Can you work these out from the model? Positions are in its coordinate system, mm. Round coordinates to 2 decimals unless told otherwise and drop trailing zeros. Write each loop counter-clockwise with the first axis right and the second up, starting at its lowest first coordinate (ties: lowest second). Pieces come first, ordered by that corner, then holes.
Q1. If we section it at C-C (y = 16): Please give me the cut outline in (x, z).
Q2. I'm going to push flat-ended pins straight in: pin 1 Ø0.7 at (y, z) = (25, 1) entering from +X; pin 2 Ø0.9 at (y, z) = (17.5, 1) entering from +X; pin 3 Ø1.6 at (x, z) = (-9, 1.5) entering from -Y. Where does each tip first touch, or does it pass through?
Q3. If we section it at A-A (y = -8): Give the number of separate pieces and of enclosed holes in the cut face, plus the area to 3 significant figures.
Q4. Please list where these lines run through material, in increasing order: line 1 along X through (y, z) = (23, 2.2); line 2 along X through (y, z) = (-12.5, 0.2); line 3 along X through (y, z) = (12.5, 2.95).
from build123d import *

# Parameters (mm, degrees)
SKETCH1_R           = 1.5
BOSS_EXTRUDE1_DEPTH = 3
SKETCH2_R           = 0.2
CUT_EXTRUDE1_DEPTH  = 51.771570482
CIRPATTERN1_COUNT   = 3
SKETCH3_R           = 8.5
CUT_EXTRUDE2_DEPTH  = 45.723637705
SKETCH4_R           = 1.5
SKETCH4_R_2         = 1.375
CUT_EXTRUDE3_DEPTH  = 45.723637705
CUT_EXTRUDE6_DEPTH  = 45.723637705
SKETCH10_R          = 1.6
BOSS_EXTRUDE3_DEPTH = 3
CUT_EXTRUDE7_DEPTH  = 46.118589611


with BuildPart() as part:
    # Sketch1 → Boss-Extrude1 (new body)
    with BuildSketch(Plane.XY):
        Polygon((8, 23), (8, 25.75), (10, 25.75), (10, 24.45), (15, 24.45), (15, 26.5), (10.5, 31), (-10.5, 31), (-15, 26.5), (-15, 24.45), (-10, 24.45), (-10, 25.75), (-8, 25.75), (-8, 23), (-8, 20.25), (-10, 20.25), (-10, 21.55), (-15, 21.55), (-15, 19.5), (-14, 18.5), (-14, 16.703779947), (-17.732948887, 10.238122813), (-21.465897773, 3.772465679), (-23.02146997, 2.874355653), (-24.387495374, 3.240381057), (-26.162847452, 2.215381057), (-23.662847452, -2.114745962), (-22.537014427, -1.464745962), (-21.537014427, -3.19679677), (-23.918584287, -4.57179677), (-26.300154147, -5.94679677), (-27.300154147, -4.214745962), (-26.174321123, -3.564745962), (-28.674321123, 0.765381057), (-30.4496732, -0.259618943), (-32.096787517, -6.40673326), (-21.596787517, -24.59326674), (-15.4496732, -26.240381057), (-13.674321123, -25.215381057), (-16.174321123, -20.885254038), (-17.300154147, -21.535254038), (-18.300154147, -19.80320323), (-15.918584287, -18.42820323), (-13.537014427, -17.05320323), (-12.537014427, -18.785254038), (-13.662847452, -19.435254038), (-11.162847452, -23.765381057), (-9.387495374, -22.740381057), (-9.02146997, -21.374355653), (-7.465897773, -20.476245627), (0, -20.476245627), (7.465897773, -20.476245627), (9.02146997, -21.374355653), (9.387495374, -22.740381057), (11.162847452, -23.765381057), (13.662847452, -19.435254038), (12.537014427, -18.785254038), (13.537014427, -17.05320323), (15.918584287, -18.42820323), (18.300154147, -19.80320323), (17.300154147, -21.535254038), (16.174321123, -20.885254038), (13.674321123, -25.215381057), (15.4496732, -26.240381057), (21.596787517, -24.59326674), (32.096787517, -6.40673326), (30.4496732, -0.259618943), (28.674321123, 0.765381057), (26.174321123, -3.564745962), (27.300154147, -4.214745962), (26.300154147, -5.94679677), (23.918584287, -4.57179677), (21.537014427, -3.19679677), (22.537014427, -1.464745962), (23.662847452, -2.114745962), (26.162847452, 2.215381057), (24.387495374, 3.240381057), (23.02146997, 2.874355653), (21.465897773, 3.772465679), (17.732948887, 10.238122813), (14, 16.703779947), (14, 18.5), (15, 19.5), (15, 21.55), (10, 21.55), (10, 20.25), (8, 20.25), align=None)
        with Locations((0, 23)):
            Circle(SKETCH1_R, mode=Mode.SUBTRACT)
        with Locations((19.918584287, -11.5)):
            Circle(SKETCH1_R, mode=Mode.SUBTRACT)
        with Locations((-19.918584287, -11.5)):
            Circle(SKETCH1_R, mode=Mode.SUBTRACT)
    extrude(amount=BOSS_EXTRUDE1_DEPTH)

    # Sketch2 → Cut-Extrude1 (cut, through all)
    with BuildSketch(Plane(origin=(8, 0, 0), x_dir=(0, 0, -1), z_dir=(1, 0, 0))):
        with Locations(Location((-1.5, 23, 0), (0, 0, 90))):
            Circle(SKETCH2_R)
    cut_extrude1 = extrude(amount=-CUT_EXTRUDE1_DEPTH, mode=Mode.SUBTRACT)

    # CirPattern1: Cut-Extrude1 ×3 about axis
    cirpattern1_axis = Axis((0, 0, -0.25), (0, 0, 1))
    for i in range(1, CIRPATTERN1_COUNT):
        add(cut_extrude1.rotate(cirpattern1_axis, i * 360 / CIRPATTERN1_COUNT), mode=Mode.SUBTRACT)

    # Sketch3 → Cut-Extrude2 (cut, through all)
    with BuildSketch(Plane.XY.offset(3)):
        Circle(SKETCH3_R)
    extrude(amount=-CUT_EXTRUDE2_DEPTH, mode=Mode.SUBTRACT)

    # Sketch4 → Cut-Extrude3 (cut, through all)
    with BuildSketch(Plane.XY.offset(3)):
        with Locations((7.5, -12.990381057)):
            Circle(SKETCH4_R)
        with Locations((-11.529543503, -3.327104841)):
            Circle(SKETCH4_R_2)
        with Locations((2.883414438, 11.648429988)):
            Circle(SKETCH4_R_2)
    extrude(amount=-CUT_EXTRUDE3_DEPTH, mode=Mode.SUBTRACT)

    # Sketch8 → Cut-Extrude6 (cut, through all)
    with BuildSketch(Plane(origin=(0, 0, 0), x_dir=(-1, 0, 0), z_dir=(0, 0, -1))):
        with BuildLine():
            Line((12.279936491, 14.683017338), (18.855834264, 3.293228289))
            ThreePointArc((18.855834264, 3.293228289), (18.94474564, 2.617879339), (18.530071655, 2.077465679))
            Line((18.530071655, 2.077465679), (14.291991324, -0.36939114))
            ThreePointArc((14.291991324, -0.36939114), (13.832521283, -0.488510893), (13.377167051, -0.354515528))
            ThreePointArc((13.377167051, -0.354515528), (8.03139394, -3.440901304), (13.566455789, -6.173328363))
            ThreePointArc((13.566455789, -6.173328363), (17.172799511, -6.424627154), (17.604766052, -10.013815228))
            ThreePointArc((17.604766052, -10.013815228), (17.57023213, -10.069006588), (17.537014427, -10.125))
            ThreePointArc((17.537014427, -10.125), (9.508411975, -15.48954065), (0.36493223, -12.38574751))
            Line((0.36493223, -12.38574751), (-6.01040764, -6.01040764))
            ThreePointArc((-6.01040764, -6.01040764), (-6.677816527, -5.258970093), (-7.251866025, -4.434009377))
            Line((-7.251866025, -4.434009377), (-18.530071655, 2.077465679))
            ThreePointArc((-18.530071655, 2.077465679), (-18.94474564, 2.617879339), (-18.855834264, 3.293228289))
            Line((-18.855834264, 3.293228289), (-12.279936491, 14.683017338))
            ThreePointArc((-12.279936491, 14.683017338), (-11.739522831, 15.097691323), (-11.064173881, 15.008779947))
            Line((-11.064173881, 15.008779947), (-8.70895574, 13.648994119))
            ThreePointArc((-8.70895574, 13.648994119), (-8.343780593, 13.24662835), (-8.280593962, 12.7069446))
            ThreePointArc((-8.280593962, 12.7069446), (-7.79681587, 9.176894763), (-5.250985835, 6.68409663))
            ThreePointArc((-5.250985835, 6.68409663), (-2.04241856, 8.250971241), (1.526575519, 8.361792104))
            ThreePointArc((1.526575519, 8.361792104), (1.938099301, 9.002110796), (2.257279563, 9.69311283))
            ThreePointArc((2.257279563, 9.69311283), (2.411493279, 9.95368058), (2.644137319, 10.147469572))
            Line((2.644137319, 10.147469572), (11.064173881, 15.008779947))
            ThreePointArc((11.064173881, 15.008779947), (11.739522831, 15.097691323), (12.279936491, 14.683017338))
        make_face()
    extrude(amount=-CUT_EXTRUDE6_DEPTH, mode=Mode.SUBTRACT)

    # Sketch10 → Boss-Extrude3 (add, through all)
    with BuildSketch(Plane(origin=(0, 0, 0), x_dir=(-1, 0, 0), z_dir=(0, 0, -1))):
        with BuildLine():
            Line((32.096787517, -6.40673326), (32.640521415, -16.833350806))
            ThreePointArc((32.640521415, -16.833350806), (31.744101835, -19.225646902), (29.382221383, -20.199386806))
            ThreePointArc((29.382221383, -20.199386806), (24.889296585, -21.332829657), (21.596787517, -24.59326674))
            Line((21.596787517, -24.59326674), (32.096787517, -6.40673326))
        make_face()
        with Locations((29.444863729, -17)):
            Circle(SKETCH10_R, mode=Mode.SUBTRACT)
    extrude(amount=-BOSS_EXTRUDE3_DEPTH)

    # Sketch11 → Cut-Extrude7 (cut, through all)
    with BuildSketch(Plane(origin=(0, 0, 0), x_dir=(-1, 0, 0), z_dir=(0, 0, -1))):
        Polygon((-4.461880215, -20.476245627), (-3.538119785, -20.476245627), (-4, -19.676245627), align=None)
    extrude(amount=-CUT_EXTRUDE7_DEPTH, mode=Mode.SUBTRACT)


solid = part.part
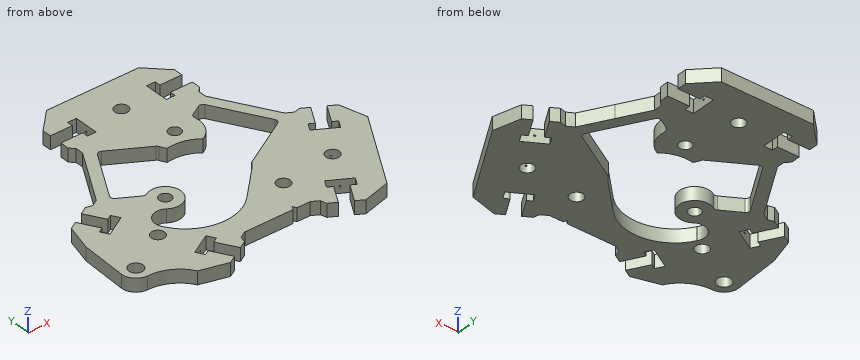
A:
1. outline: (-14.41, 0) - (14.41, 0) - (14.41, 3) - (-14.41, 3) - close
2. pin 1: stops at x = 15
2. pin 2: stops at x = 14
2. pin 3: stops at y = -22.98
3. separate pieces: 2
3. enclosed holes: 2
3. area: 124 mm2
4. line 1: x = -8 to -1.5, 1.5 to 8
4. line 2: x = -32.41 to -21.04, -18.8 to -15.69, -0.48 to 6.08, 8.92 to 18.8, 21.04 to 28.58
4. line 3: x = -16.43 to -13.54, -6.72 to 1.8, 3.96 to 8.32, 13.54 to 16.43
